Verification items for this drawing (mm, ordinates from the low corner). A direction names the side the tool comes from. Give positions to 0.01 mm unless a question says otherwise; leave off trailing zeros. Write each loop counter-clockwise with the first axis right and the second up, starting at its lowest first coordinate (ties: lowest second). Pieces come first, ordered by that corner, then holes. Notation, with made-up numbers: (-31.5, 46) -> (1.5, 46) arc R25 ccw to (1.5, 62) -> close; hole circle Ø11 at (52.5, 47). An arc over 180 degrees is marked (long way). Answer as a JSON object with one key per item and string values.
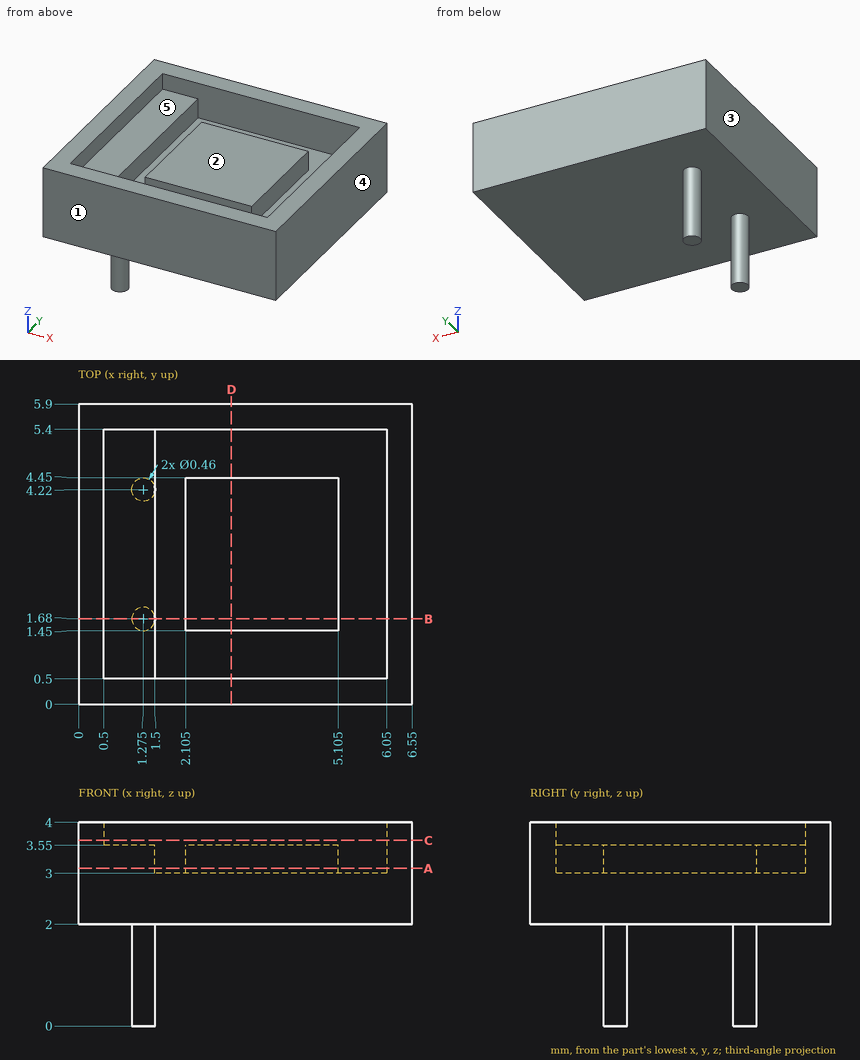
1. Mould release check, pull along X, two halves, no side actions. Record for the marked faces 1, 2 and 3: released by +X, released by -X, zero draft, split by the parting line, or undercut.
Determined:
{"face 1": "zero draft", "face 2": "undercut", "face 3": "released by -X"}
2. Sectioned sample at A-A, the plane z = 3.1. Enter the section's corners in (x, y) (3 decimals).
Determined:
{"outline": "(0, 0) -> (6.55, 0) -> (6.55, 5.9) -> (0, 5.9) -> close; (2.105, 1.45) -> (5.105, 1.45) -> (5.105, 4.45) -> (2.105, 4.45) -> close; hole (1.5, 0.5) -> (6.05, 0.5) -> (6.05, 5.4) -> (1.5, 5.4) -> close"}
3. Scan lines: L1, parallel to Z at x = 6, y = 4.85; L2, parallel to Z at x = 2.5, y = 3.35; L3, parallel to X at y = 1.4, z = 3.3. Record each from-to range of solid material in increasing order. Write a range as [from, to].
Determined:
{"L1": "[2, 3]", "L2": "[2, 3.55]", "L3": "[0, 1.5], [6.05, 6.55]"}
4. Sectioned sample at D-D, the plane x = 3. Enter the section's corners in (y, z).
Determined:
{"outline": "(0, 2) -> (5.9, 2) -> (5.9, 4) -> (5.4, 4) -> (5.4, 3) -> (4.45, 3) -> (4.45, 3.55) -> (1.45, 3.55) -> (1.45, 3) -> (0.5, 3) -> (0.5, 4) -> (0, 4) -> close"}
5. Go/stop test with flat-tipped pins: P1, Ø0.9, axis at x = 4, y = 3, coming from the +Z side; P2, Ø1.5, axis at x = 3.5, y = 2, coming from the -Z side. Record where each tip stops, or that it passes through.
Determined:
{"P1": "z = 3.55", "P2": "z = 2"}
6. Access from +Z, -Z, +X, -X, +Y, -Y to the whole of each face (thin tool, end or side, straight path). Record for the marked faces 4 and 5.
Determined:
{"face 4": "+Z, -Z, +X, +Y, -Y", "face 5": "+Z"}
7. Sectioned sample at C-C, the plane z = 3.65. Enter the section's corners in (x, y), plus the area to 4 significant figures.
Determined:
{"outline": "(0, 0) -> (6.55, 0) -> (6.55, 5.9) -> (0, 5.9) -> close; hole (0.5, 0.5) -> (6.05, 0.5) -> (6.05, 5.4) -> (0.5, 5.4) -> close", "area": "11.45 mm^2"}
8. Sectioned sample at B-B, the plane y = 1.68. Enter the section's corners in (x, z) (3 decimals).
Determined:
{"outline": "(0, 2) -> (1.045, 2) -> (1.045, 0) -> (1.505, 0) -> (1.505, 2) -> (6.55, 2) -> (6.55, 4) -> (6.05, 4) -> (6.05, 3) -> (5.105, 3) -> (5.105, 3.55) -> (2.105, 3.55) -> (2.105, 3) -> (1.5, 3) -> (1.5, 3.55) -> (0.5, 3.55) -> (0.5, 4) -> (0, 4) -> close"}
